from build123d import *

# Parameters (mm, degrees)
F0_W         = 48.5600655451
F0_H         = 43.9142854884
F0_W_2       = 42.5600655451
F0_H_2       = 37.9142854884
F1_DEPTH     = 127
F2_DEPTH     = 3
F3_R         = 5
F4_T1_DEPTH  = 51.7727004283
F4_T3_DEPTH  = 69.6311153681
F4_T5_DEPTH  = 74.2768954248
F4_T7_DEPTH  = 56.418480485
F4_T10_ANGLE = 90
F5_R         = 5
F6_SIZE      = 5


# Not quite as in the source:
# - a fillet or chamfer that OpenCascade refuses, or shapes differently, is made with other operations: its cross-section is extruded or revolved along the edge and cut away or added


with BuildPart() as f1:
    # F0 (on Top) → F1 (new body)
    with BuildSketch(Plane.XY):
        with Locations((13.9204316549, -10.4247569107)):
            Rectangle(F0_W, F0_H)
        with Locations((13.9204316549, -10.4247569107)):
            Rectangle(F0_W_2, F0_H_2, mode=Mode.SUBTRACT)
    extrude(amount=-F1_DEPTH)

    # F0 (on Top) → F2 (join)
    with BuildSketch(Plane.XY):
        with Locations((13.9204316549, -10.4247569107)):
            Rectangle(F0_W_2, F0_H_2)
    extrude(amount=-F2_DEPTH)

    # F3
    f3_edges = [f1.edges().sort_by_distance(p)[0] for p in [
        (-10.359601, -32.3819, -63.5),
    ]]
    fillet(f3_edges, radius=F3_R)

    # F4: chamfer of 5 on 3 edges, made by hand

    # F4_s2 → F4_t1 (cut)
    with BuildSketch(Plane.XZ.offset(-24.3908007734)):
        Polygon((-10.3596011177, -122), (-5.3596011177, -127), (-10.3596011177, -127), align=None)
    extrude(amount=F4_T1_DEPTH, mode=Mode.SUBTRACT)

    # F4_s4 → F4_t3 (cut)
    with BuildSketch(Plane.XZ.offset(-24.3908007734)):
        Polygon((33.2004644275, -127), (38.2004644275, -122), (38.2004644275, -127), align=None)
    extrude(amount=F4_T3_DEPTH, mode=Mode.SUBTRACT)

    # F4_s6 → F4_t5 (cut)
    with BuildSketch(Plane.YZ.offset(-23.2180160575)):
        Polygon((11.5323858336, -122), (6.5323858336, -127), (11.5323858336, -127), align=None)
    extrude(amount=F4_T5_DEPTH, mode=Mode.SUBTRACT)

    # F4_s8 → F4_t7 (cut)
    with BuildSketch(Plane.YZ.offset(-5.3596011177)):
        Polygon((-27.3818996549, -127), (-32.3818996549, -122), (-32.3818996549, -127), align=None)
    extrude(amount=F4_T7_DEPTH, mode=Mode.SUBTRACT)

    # F4_s9 → F4_t10 (revolve, cut)
    with BuildSketch(Plane.XZ.offset(27.3818996549)):
        Polygon((-10.3596011177, -122), (-5.3596011177, -127), (-10.3596011177, -127), align=None)
    revolve(axis=Axis((-5.3596011177, -27.3818996549, -127), (0, 0, 1)), revolution_arc=F4_T10_ANGLE, mode=Mode.SUBTRACT)

    # F5
    f5_edges = [f1.edges().sort_by_distance(p)[0] for p in [
        (-10.359601, 11.532386, -61),
        (38.200464, 11.532386, -61),
        (38.200464, -32.3819, -61),
    ]]
    fillet(f5_edges, radius=F5_R)

    # F6
    f6_edges = [f1.edges().sort_by_distance(p)[0] for p in [
        (13.920432, -32.3819, 0),
    ]]
    chamfer(f6_edges, length=F6_SIZE)


solid = f1.part
The model under review builds one solid part; all positions refer to its coordinate system, in mm. Round coordinates to 2 decimals unless told otherwise and drop trailing zeros. Loops run counter-clockwise (first coordinate to the right, second up) from the corner with the lowest first, then second, coordinate; pieces in that order, holes last. Notation, with made-up numbers: (3.25, 82.25) -> (54.25, 82.25) arc R22 cw to (54.25, 115.25) -> close; hole circle Ø7 at (32, -20). An arc over 180 degrees is marked (long way). Write item = value, one per line. Start each with the question number.
Item 1: To check wall thickness, follow L1, parallel to Y at x = -3.5, z = -101; L2, parallel to X at y = -20, z = -119; L3, parallel to Z at x = 15, y = 0.5. State the ranges of each line that lie inside material, in increasing order.
Item 2: Take a section at A-A on z = -36. Give the boundary of the cut face in (x, y).
Item 3: Take a section at B-B on x = 23.5. Give the boundary of the cut face in (y, z), plus the area to 3 significant figures.
Item 4: Mouldability with a two-part tool opening along X and no side actions: class faces 1 (the flat face through (14, 8.532, -63)), 2 (the flat face through (-7.36, -11, -63)), 3 (the flat face through (35.7, -10.7, -2.5)), 4 (the flat face through (14, -32.382, -63)) as released by +X, released by -X, zero draft, split by the parting line, or undercut.
Item 5: Take a section at C-C on y = -0.5. Give the boundary of the cut face in (x, z), plus the area to 3 significant figures.
Item 6: Insertion check: pin 1 (12 mm diameter, centred on x = 27.5, y = -23, fed in from -Z). The pin has a flat end and moves straight along its axis. Give the tip position at first contact, or say it passes through.
Result:
q1.L1 = -32.38 to -29.38, 8.53 to 11.53
q1.L2 = -10.36 to -7.36, 35.2 to 38.2
q1.L3 = -3 to 0
q2.outline = (-10.36, -27.38) arc R5 ccw to (-5.36, -32.38) -> (33.2, -32.38) arc R5 ccw to (38.2, -27.38) -> (38.2, 6.53) arc R5 ccw to (33.2, 11.53) -> (-5.36, 11.53) arc R5 ccw to (-10.36, 6.53) -> close; hole (-7.36, -29.38) -> (35.2, -29.38) -> (35.2, 8.53) -> (-7.36, 8.53) -> close
q3.outline = (-32.38, -122) -> (-29.38, -125) -> (-29.38, -3) -> (8.53, -3) -> (8.53, -125) -> (11.53, -122) -> (11.53, -5) -> (6.53, 0) -> (-27.38, 0) -> (-32.38, -5) -> close
q3.area = 830 mm²
q4.face_1 = undercut
q4.face_2 = undercut
q4.face_3 = released by +X
q4.face_4 = zero draft
q5.outline = (-10.36, -122) -> (-7.36, -125) -> (-7.36, -3) -> (35.2, -3) -> (35.2, -125) -> (38.2, -122) -> (38.2, -5) -> (33.2, 0) -> (-5.36, 0) -> (-10.36, -5) -> close
q5.area = 844 mm²
q6.pin_1 = -3
